Study the drawing (mm; zero at the part's minimum x, y, z) and answer. A direction names the side the tool comes from. Coordinates: 2 decimals unless noted, no trailing zeros. Order: outer loops, then holes, each group sorted by start corner. A loop starts at its lowest first (then second) coordinate and runs counter-clockwise, first axis right, second up.
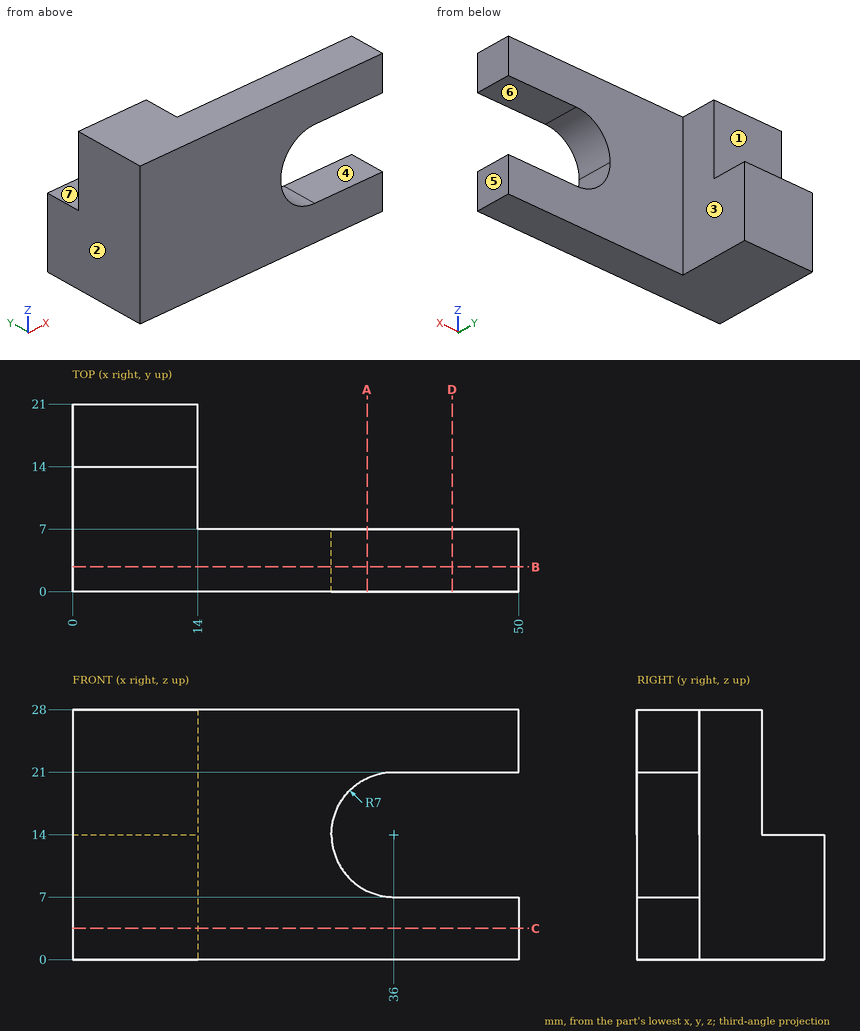
(1) Find section C-C on z = 3.5. Determine the outline of the cut face in (x, y), then the cut area to 3 significant figures.
(2) Find section D-D on x = 42.5. Determine the outline of the cut face in (y, z), then the cut area to 3 significant figures.
(3) Given pin 1 Ø7 at (y, z) = (13.5, 15) entering from +X; pin 2 Ø5 at (x, z) = (26, 4.5) entering from +Y; pin 3 Ø3 at (x, z) = (34.5, 10.5) entering from +Y; pin 4 Ø7 at (x, z) = (5.5, 24) entering from +Y, each flat-ended and moving along its own axis, determine where each tip first touches the part or whether it passes through.
(4) Find section A-A on x = 33. Determine the outline of the cut face in (y, z), then the cut area to 3 significant figures.
(5) A tool of negligible diameter and unlimited length cuts with its end or side. For the marked faces 1, 2 and 3, from which of +Z, -Z, +X, -X, +Y, -Y can it reach the whole face along a straight path? Write none if from no direction.
(6) Find the intervals of material crossed by probe 1 along X at (y, z) = (8.75, 12.75); probe 2 along Y at (x, z) = (39.5, 6.5), in increasing order.
(7) Find section B-B on y = 2.75. Determine the outline of the cut face in (x, z), then the cut area to 3 significant figures.
(8) The mould has two halves that part along Z. Classify the marked faces 4, 5, 6 and 7: pulls with the +Z half, pulls with the -Z half, needs draft (parallel to the pull), parting line crosses it, or undercut.
Resolved:
1. outline: (0, 0) - (50, 0) - (50, 7) - (14, 7) - (14, 21) - (0, 21) - close
1. area: 546 mm2
2. outline: (0, 0) - (7, 0) - (7, 7) - (0, 7) - close; (0, 21) - (7, 21) - (7, 28) - (0, 28) - close
2. area: 98.0 mm2
3. pin 1: stops at x = 14
3. pin 2: stops at y = 7
3. pin 3: passes through
3. pin 4: stops at y = 14
4. outline: (0, 0) - (7, 0) - (7, 7.68) - (0, 7.68) - close; (0, 20.32) - (7, 20.32) - (7, 28) - (0, 28) - close
4. area: 107 mm2
5. face 1: +Z, +X, -X, +Y
5. face 2: +Z, -Z, -X, +Y, -Y
5. face 3: +Z, -Z, +X, +Y
6. probe 1: x = 0 to 14
6. probe 2: y = 0 to 7
7. outline: (0, 0) - (50, 0) - (50, 7) - (36, 7) arc R7 cw to (36, 21) - (50, 21) - (50, 28) - (0, 28) - close
7. area: 1,130 mm2
8. face 4: undercut
8. face 5: needs draft
8. face 6: undercut
8. face 7: pulls with the +Z half
